Check sheet for the modelled part. Datum: model origin and axes. Units: mm. A direction names the side the tool comes from. Give positions to 0.01 mm unless a question says otherwise; leave off trailing zeros. Write each loop counter-clockwise with the first axis right and the second up, starting at its lowest first coordinate (ties: lowest second). Pieces come first, ordered by that corner, then holes. Notation, with made-up numbers: (79, -33.75) -> (99, -33.75) arc R5 cw to (99, -27.75) -> close; hole circle Ø3 at (-2.5, 67). An arc over 180 degrees is marked (long way). Write each question's results on one line, items separated by ' | '. Start each with the question number.
```python
from build123d import *


with BuildPart() as part:
    # Sketch1 → Revolve1 (revolve)
    with BuildSketch(Plane.XY):
        with BuildLine():
            Line((9.75, 0), (10.875, 0))
            ThreePointArc((10.875, 0), (11.582106781, 0.292893219), (11.875, 1))
            Line((11.875, 1), (11.875, 46.5))
            ThreePointArc((11.875, 46.5), (10.593592168, 49.593592168), (7.5, 50.875))
            Line((7.5, 50.875), (7.75, 50.875))
            Line((7.75, 50.875), (7.75, 52.875))
            Line((7.75, 52.875), (10, 52.875))
            Line((10, 52.875), (10, 69.075))
            Line((10, 69.075), (8.15, 69.075))
            Line((8.15, 69.075), (8.15, 77.275))
            Line((8.15, 77.275), (7.2, 77.275))
            Line((7.2, 77.275), (7.2, 89.975))
            Line((7.2, 89.975), (0, 89.975))
            Line((0, 89.975), (0, 65.8))
            Line((0, 65.8), (0, 2.409558552))
            Line((0, 2.409558552), (7.75, 2.409558552))
            ThreePointArc((7.75, 2.409558552), (8.457106781, 2.116665333), (8.75, 1.409558552))
            Line((8.75, 1.409558552), (8.75, 1))
            ThreePointArc((8.75, 1), (9.042893219, 0.292893219), (9.75, 0))
        make_face()
    revolve(axis=Axis((0, 65.8, 0), (0, -1, 0)))


solid = part.part
```
Item 1: Set-up check for faces 4 (the flat face through (0, 2.41, 0)), 5 (the flat face through (-2.9, 52.875, -7.4)), 6 (the flat face through (2, 0, 10)), 7 (the cylindrical face through (-2.574, 24.068, -11.593)), 8 (the flat face through (-3.8, 69.075, -7.4)): record each of +Z, -Z, +X, -X, +Y, -Y from which the full face is reachable in a straight line by a thin tool's end or side.
Item 2: Mould release check, pull along X, two halves, no side actions. Record for faces 1 (the cylindrical face through (-6.944, 1.202, -5.324)), 2 (the flat face through (3, 77.275, -7)), 3 (the cylindrical face through (-6.468, 73.232, -4.959)): pulls with the +X half, pulls with the -X half, needs draft (parallel to the pull), parting line crosses it, or undercut.
Item 3: Depth check by flat-ended pin: pin 1 Ø12.5 at (x, z) = (-2, 2) entering from -Y; pin 2 Ø6 at (y, z) = (57, 8.5) entering from +X; pin 3 Ø12.5 at (x, z) = (-0.5, 1) entering from -Y. Enter the tip coordinate at first touch or a pass-through.
Item 4: Section check C-C on y = 26. Record the boundary of the cut face in (x, z) (3 decimals), then the cut area to 3 significant figures.
Item 5: Thickness scan on probe 1 along Z at (x, y) = (0, 1.2) (3 decimals); probe 2 along Y at (x, z) = (0.25, 4.5) (3 decimals); probe 3 along Z at (x, y) = (-9, 38). Record the ranges inside material, lowest first. Write a range as from..to.
Check sheet entries:
1) face 4: -Y | face 5: none | face 6: +Z, -Z, +X, -X, -Y | face 7: +Y, -Y | face 8: +Y
2) face 1: undercut | face 2: needs draft | face 3: parting line crosses it
3) pin 1: stops at y = 0.26 | pin 2: stops at x = 8.35 | pin 3: stops at y = 2.41
4) outline: circle Ø23.75 at (0, 0) | area: 443 mm^2
5) probe 1: z = -11.875..-8.75, 8.75..11.875 | probe 2: y = 2.41..89.975 | probe 3: z = -7.75..7.75
